Autodesk Inventor part; units mm, degrees
ref_plane "YZ Plane" through (0, 0, 0) normal (1, 0, 0) x (0, 1, 0)
ref_plane "XZ Plane" through (0, 0, 0) normal (0, 1, 0) x (-1, 0, 0)
ref_plane "XY Plane" through (0, 0, 0) normal (0, 0, 1) x (1, 0, 0)
sketch "Sketch1" plane through (0, 0, 0) normal (0, 0, 1) x (1, 0, 0)
  line L0 (0, 0) -> (3.175, 0)
  line L1 (3.175, 0) -> (3.175, -3.175)
  line L2 (3.175, -3.175) -> (15.875, -3.175)
  line L3 (15.875, -3.175) -> (15.875, 0)
  line L4 (0, 0) -> (0, 25.4)
  line L5 (307.975, 0) -> (15.875, 0)
  line L6 (0, 25.4) -> (-11.8442, 50.8)
  line L7 (307.975, 25.4) -> (263.9809, 50.8)
  line L8 (-11.8442, 50.8) -> (263.9809, 50.8)
  line L9 (358.775, 0) -> (422.275, 0)
  line L10 (307.975, 0) -> (358.775, 0)
  line L11 (307.975, 25.4) -> (384.175, 25.4)
  line L12 (384.175, 241.3) -> (422.275, 241.3)
  line L13 (588.0391, 190.1261) -> (586.2287, 190.1261)
  line L14 (586.2287, 218.7011) -> (586.2287, 190.1261)
  line L15 (588.0391, 218.7011) -> (586.2287, 218.7011)
  line L16 (588.0391, 190.1261) -> (588.0391, 218.7011)
  line L17 (588.0391, 38.1) -> (586.2287, 38.1)
  line L18 (586.2287, 177.4261) -> (586.2287, 38.1)
  line L19 (586.2287, 177.4261) -> (588.0391, 177.4261)
  line L20 (588.0391, 38.1) -> (588.0391, 177.4261)
  line L21 (588.0391, 190.1261) -> (588.0391, 218.7011)
  line L22 (588.0391, 190.1261) -> (586.2287, 190.1261)
  line L23 (586.2287, 218.7011) -> (586.2287, 190.1261)
  line L24 (588.0391, 218.7011) -> (586.2287, 218.7011)
  line L25 (588.0391, 190.1261) -> (588.0391, 218.7011)
  line L26 (431.5435, 218.7011) -> (431.5435, 12.7)
  line L27 (431.5435, 218.7011) -> (429.7331, 218.7011)
  line L28 (429.7331, 12.7) -> (429.7331, 218.7011)
  line L29 (431.5435, 12.7) -> (429.7331, 12.7)
  line L30 (384.175, 25.4) -> (422.275, 25.4)
  line L31 (422.275, 0) -> (422.275, 25.4)
  dimension "d0" = 3.175
  dimension "d1" = 3.175
  dimension "d2" = 12.7
  dimension "d3" = 25.4
  dimension "d4" = 307.975
  dimension "d12" = 25.4
  dimension "d13" = 25
  dimension "d17" = 25.4
  dimension "d19" = 150
  dimension "d21" = 25.4
  dimension "d25" = 0
  dimension "d36" = 215.9
  dimension "d37" = 38.1
  dimension "d44" = 76.2
extrude "Extrusion1" add sketch "Sketch1" along normal blind 3.175 contours L4 L6 L8 L7 L11 L30 L31 L9 L10 L5 L3 L2 L1 L0
sketch "Sketch2" plane through (0, 0, 3.175) normal (0, 0, 1) x (1, 0, 0)
  line L0 (289.5902, 0) -> (302.2902, 0)
  line L1 (289.5902, -3.175) -> (289.5902, 0)
  line L2 (302.2902, -3.175) -> (289.5902, -3.175)
  line L3 (302.2902, 0) -> (302.2902, -3.175)
extrude "Extrusion2" add sketch "Sketch2" against normal blind 3.175
sketch "Sketch6" plane through (0, 0, 0) normal (0, 0, -1) x (-1, 0, 0)
  line L0 (-422.275, 0) -> (-422.275, 50.8)
  line L1 (-422.275, 0) -> (-473.075, 29.3294)
  line L2 (-462.0765, 48.3794) -> (-422.275, 25.4)
  line L3 (-473.075, 29.3294) -> (-462.0765, 48.3794)
  point P0 (-407.9875, 50.8)
  dimension "d53" = 60
extrude "Extrusion6" add sketch "Sketch6" against normal blind 3.175
sketch "Sketch7" plane through (0, 0, 0) normal (0, 0, -1) x (-1, 0, 0)
  line L0 (-473.075, 29.3294) -> (-422.275, 0)
  line L1 (-3.175, 0) -> (-3.175, -3.175)
  line L2 (-422.275, 0) -> (-438.15, 0)
  line L3 (-438.15, 0) -> (-477.0438, 22.4553)
  line L4 (-473.075, 29.3294) -> (-477.0438, 22.4553)
  dimension "d58" = 15.875
extrude "Extrusion7" add sketch "Sketch7" against normal blind 3.175
sketch "Sketch8" plane through (0, 0, 0) normal (0, 0, -1) x (-1, 0, 0)
  line L0 (-422.275, 25.4) -> (-462.0765, 48.3794)
  line L1 (-477.0438, 22.4553) -> (-438.15, 0)
  line L2 (-422.275, 25.4) -> (-403.225, 58.3956)
  line L3 (-462.0765, 48.3794) -> (-443.0265, 81.375)
  line L4 (-443.0265, 81.375) -> (-403.225, 58.3956)
  dimension "d61" = 38.1
  dimension "d62" = 38.1
extrude "Extrusion8" add sketch "Sketch8" against normal blind 3.175
sketch "Sketch9" plane through (0, 0, 3.175) normal (0, 0, 1) x (1, 0, 0)
  line L0 (0, 0) -> (3.175, 0)
  line L1 (3.175, 0) -> (3.175, -3.175)
  line L2 (3.175, -3.175) -> (15.875, -3.175)
  line L3 (15.875, -3.175) -> (15.875, 0)
  line L4 (15.875, 0) -> (289.5902, 0)
  line L5 (289.5902, 0) -> (289.5902, -3.175)
  line L6 (289.5902, -3.175) -> (302.2902, -3.175)
  line L7 (302.2902, -3.175) -> (302.2902, 0)
  line L8 (302.2902, 0) -> (438.15, 0)
  line L9 (438.15, 0) -> (477.0438, 22.4553)
  line L10 (477.0438, 22.4553) -> (443.0265, 81.375)
  line L11 (443.0265, 81.375) -> (403.225, 58.3956)
  line L12 (403.225, 58.3956) -> (422.275, 25.4)
  line L13 (422.275, 25.4) -> (307.975, 25.4)
  line L14 (307.975, 25.4) -> (263.9809, 50.8)
  line L15 (263.9809, 50.8) -> (-11.8442, 50.8)
  line L16 (-11.8442, 50.8) -> (0, 25.4)
  line L17 (0, 25.4) -> (0, 0)
properties part number "Side Wall 2" material "Polycarbonate, Clear"
Here's how the part is built. I have some questions about the finished solid (model axes, mm). Give positions to 0.01 mm unless a question says otherwise; leave off trailing zeros. Order: outer loops, then holes, each group sorted by start corner. A loop starts at its lowest first (then second) coordinate and runs counter-clockwise, first axis right, second up. Notation, with made-up numbers: (32.25, 40) -> (77.25, 40) arc R20 cw to (77.25, 52) -> close; hole circle Ø3 at (73, 51). An arc over 180 degrees is marked (long way). One line per item, written item: value. Start each with the question number.
1. Imagine slicing it at C-C, the plane x = 136. List the corners of the cut face in (y, z) for me (3 decimals).
2. We'd pull the mould along X, two halves only. Please class faces 1 (the face through (286.29, 37.92, 1.57)), 2 (the face through (457.32, 11.07, 1.57)), 3 (the face through (412.88, 41.67, 1.57)), 4 (the face through (-5.84, 37.92, 1.57)): released by +X, released by -X, zero draft, split by the parting line, or undercut.
3. Imagine slicing it at A-A, the plane y = 37.5. List the corners of the cut face in (x, z) for me (3 decimals).
4. Imagine slicing it at D-D, the plane y = 13. List the corners of the cut face in (x, z) for me (3 decimals).
5. I need wall thicknesses on probe 1 along Y at (x, z) = (378.5, 2.35); probe 2 along X at (y, z) = (49.5, 0.2); probe 3 along Y at (x, z) = (208.5, 2.7). Which ranges of each line are inside material? Lowest first, please. Write a range as from..to.
6. Will these pins go through, and if not, where does the flat tip stop? pin 1 Ø1 at (x, z) = (340.5, 2) entering from +Y; pin 2 Ø1.6 at (x, z) = (168, 1) entering from -Y; pin 3 Ø1 at (y, z) = (62.5, 2.5) entering from -X.
Values follow:
1. outline: (0, 0) -> (50.8, 0) -> (50.8, 3.175) -> (0, 3.175) -> close
2. face 1: undercut
2. face 2: released by +X
2. face 3: undercut
2. face 4: released by -X
3. outline: (-5.642, 0) -> (287.017, 0) -> (287.017, 3.175) -> (-5.642, 3.175) -> close; (415.289, 0) -> (468.358, 0) -> (468.358, 3.175) -> (415.289, 3.175) -> close
4. outline: (0, 0) -> (460.667, 0) -> (460.667, 3.175) -> (0, 3.175) -> close
5. probe 1: y = 0..25.4
5. probe 2: x = -11.24..266.23, 408.36..461.43
5. probe 3: y = 0..50.8
6. pin 1: stops at y = 25.4
6. pin 2: stops at y = 0
6. pin 3: stops at x = 409.47
